from build123d import *

# Parameters (mm, degrees)
EXTRUDE_1_DEPTH     = 3
SKETCH_4_W          = 13
SKETCH_4_H          = 4
CUT_EXTRUDE_1_DEPTH = 62.023006498


with BuildPart() as part:
    # 草图2 → 凸台-拉伸1 (new body)
    with BuildSketch(Plane(origin=(0, 0, 0), x_dir=(1, 0, 0), z_dir=(0, 1, 0))):
        with BuildLine():
            Line((17.732480436, 10.381771038), (-57.267519564, 10.381771038))
            Line((-57.267519564, 10.381771038), (-57.267519564, -9.618228962))
            Line((-57.267519564, -9.618228962), (43.922480436, -9.618228962))
            Line((43.922480436, -9.618228962), (43.922480436, 10.381771038))
            Line((43.922480436, 10.381771038), (20.060175686, 10.381771038))
            add(Edge.make_bspline(
                [(17.732480436, 10.381771038), (18.54587785, 10.302233399), (19.322070314, 10.305337221), (20.060175686, 10.381771038)],
                knots=[0, 0, 0, 0, 0.115465336, 0.115465336, 0.115465336, 0.115465336], degree=3))
        make_face()
        with BuildLine():
            add(Edge.make_bspline(
                [(20.060175686, 10.381771038), (25.714511546, 10.96730054), (29.13370972, 15.856194464), (29.921192775, 20.862370643)],
                knots=[0.115465336, 0.115465336, 0.115465336, 0.115465336, 1, 1, 1, 1], degree=3))
            Line((20.060175686, 10.381771038), (43.922480436, 10.381771038))
            Line((43.922480436, 10.381771038), (43.921192775, 20.862370643))
            Line((43.921192775, 20.862370643), (29.921192775, 20.862370643))
        make_face()
    extrude(amount=EXTRUDE_1_DEPTH)

    # 草图4 → 切除-拉伸1 (cut, through all)
    with BuildSketch(Plane(origin=(0, 3, 0), x_dir=(1, 0, 0), z_dir=(0, 1, 0))):
        with Locations((22.312601946, -0.100962334)):
            Rectangle(SKETCH_4_W, SKETCH_4_H)
    extrude(amount=-CUT_EXTRUDE_1_DEPTH, mode=Mode.SUBTRACT)


solid = part.part
Geometry check sheet. Reference: the model listing, model coordinates, mm. A direction names the side the tool comes from. Coordinates: 2 decimals unless noted, no trailing zeros. Order: outer loops, then holes, each group sorted by start corner. A loop starts at its lowest first (then second) coordinate and runs counter-clockwise, first axis right, second up. Notation, with made-up numbers: (54, -38) - (61, -38) arc R25 cw to (61, -4) - close; hole circle Ø5 at (36.25, 70.25). An arc over 180 degrees is marked (long way). One line per item, written item: value.
(1) Sectioned sample at B-B (x = -23.5). Enter the section's corners in (y, z), and give its area (3 significant figures).
Data:
outline: (0, -10.38) - (3, -10.38) - (3, 9.62) - (0, 9.62) - close
area: 60.0 mm^2
(2) Sectioned sample at A-A (z = -0.5). Enter the section's corners in (x, y), and give its area (3 significant figures).
Data:
outline: (-57.27, 0) - (15.81, 0) - (15.81, 3) - (-57.27, 3) - close; (28.81, 0) - (43.92, 0) - (43.92, 3) - (28.81, 3) - close
area: 265 mm^2
(3) Depth check by flat-ended pin: pin 1 Ø10 at (x, z) = (-27, -2) entering from -Y; pin 2 Ø6 at (x, z) = (-28.5, -16) entering from +Y; pin 3 Ø0.9 at (x, y) = (-19, 1.5) entering from -Z. Enter the tip coordinate at first touch or a pass-through.
Data:
pin 1: stops at y = 0
pin 2: passes through
pin 3: stops at z = -10.38
(4) Thickness scan on probe 1 along X at (y, z) = (2, 1.5); probe 2 along Z at (x, y) = (18.5, 1); probe 3 along Z at (x, y) = (23.5, 0.5). Record the ranges inside material, lowest first. Write a range as from..to.
Data:
probe 1: x = -57.27..15.81, 28.81..43.92
probe 2: z = -10.33..-1.9, 2.1..9.62
probe 3: z = -11.37..-1.9, 2.1..9.62
(5) Access from +Z, -Z, +X, -X, +Y, -Y to the whole of each face (thin tool, end or side, straight path). Record for faces 1 (the face through (-57.268, 1, -1)), 2 (the face through (-19, 1, -10.382)), 3 (the face through (15.813, 2, 0)).
Data:
face 1: +Z, -Z, -X, +Y, -Y
face 2: -Z, -X, +Y, -Y
face 3: +Y, -Y
